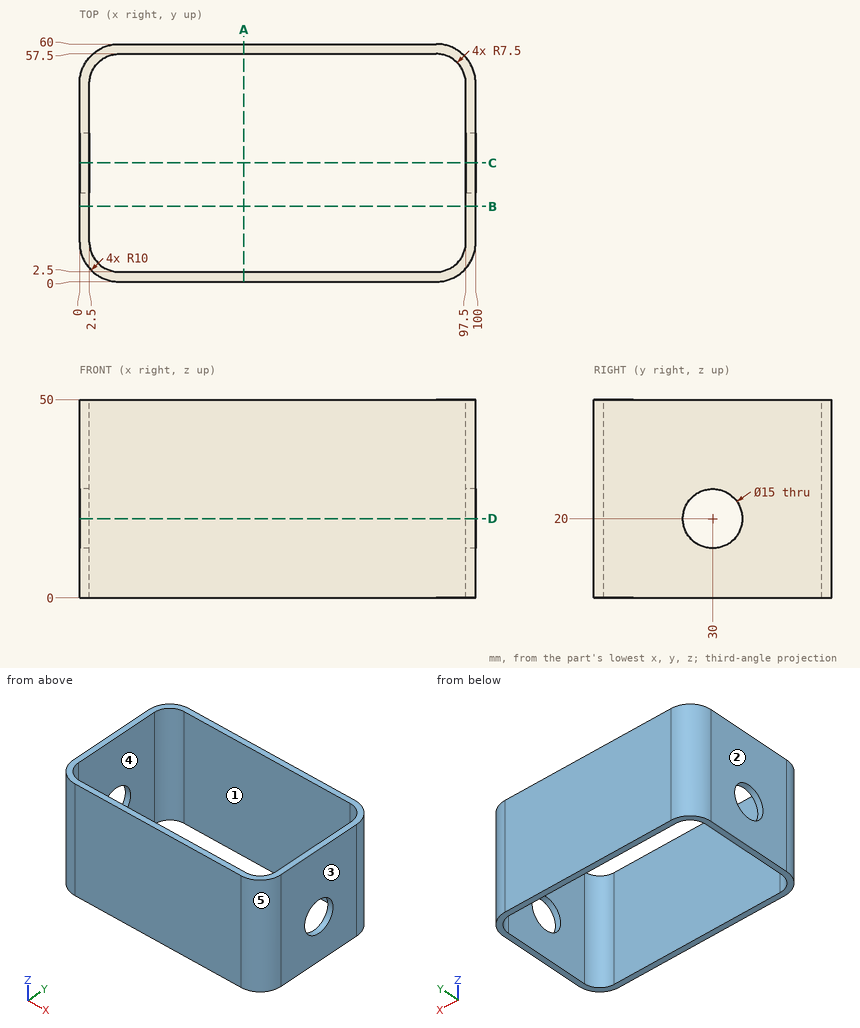
Input: dimensioned drawing with shaded views. Units: mm. Origin: part minimum x, y, z. A direction names the side the tool comes from. Give positions to 0.01 mm unless a question says otherwise; leave off trailing zeros. Loops run counter-clockwise (first coordinate to the right, second up) from the corner with the lowest first, then second, coordinate; pieces in that order, holes last. Notation, with made-up numbers: M 16.5,30.5 L 48.5,30.5 A16 ccw 48.5,47.5 Z; hole C -11.5,39 d3. An arc over 180 degrees is marked long. Put each result on its own line as item: value.
1) Cut plane C-C, the plane y = 30. Return the cut outline in (x, z), plus the area to 3 significant figures.
Computed values:
outline: M 0,0 L 2.5,0 L 2.5,12.5 L 0,12.5 Z; M 0,27.5 L 2.5,27.5 L 2.5,50 L 0,50 Z; M 97.5,0 L 100,0 L 100,12.5 L 97.5,12.5 Z; M 97.5,27.5 L 100,27.5 L 100,50 L 97.5,50 Z
area: 175 mm^2
2) Cut plane B-B, the plane y = 19. Return the cut outline in (x, z), plus the area to 3 significant figures.
Computed values:
outline: M 0,0 L 2.5,0 L 2.5,50 L 0,50 Z; M 97.5,0 L 100,0 L 100,50 L 97.5,50 Z
area: 250 mm^2
3) First-contact query: P1, Ø12, axis at y = 30, z = 20, coming from the +X side; P2, Ø5, axis at y = 6, z = 39.5, coming from the +X side. Flat tips, straight axial feed; report the tip coordinate or a pass-through.
Computed values:
P1: passes through
P2: stops at x = 99.89
4) Mould query, pull axis X, two halves, no side actions, for the marked faces 1, 2 and 3. Classes: released by +X, released by -X, zero draft, split by the parting line, or undercut.
Computed values:
face 1: undercut
face 2: released by -X
face 3: released by +X
5) Material intervals for L1, parallel to X at y = 13, z = 32; L2, parallel to Y at x = 62, z = 20; L3, parallel to Z at x = 99.15, y = 30, sorted ascending. Write a range as from..to.
Computed values:
L1: x = 0..2.5, 97.5..100
L2: y = 0..2.5, 57.5..60
L3: z = 0..12.5, 27.5..50
6) Reachability of the marked faces 4 and 5 from +Z, -Z, +X, -X, +Y, -Y: full face, straight path, thin tool, end or side. Return the list, or none.
Computed values:
face 4: +Z, -Z
face 5: +Z, -Z, +X, -Y
7) Cut plane A-A, the plane x = 41.5. Return the cut outline in (y, z).
Computed values:
outline: M 0,0 L 2.5,0 L 2.5,50 L 0,50 Z; M 57.5,0 L 60,0 L 60,50 L 57.5,50 Z
8) Cut plane D-D, the plane z = 20. Return the cut outline in (x, y), plus the area to 3 significant figures.
Computed values:
outline: M 0,10 A10 ccw 10,0 L 90,0 A10 ccw 100,10 L 100,22.5 L 97.5,22.5 L 97.5,10 A7.5 cw 90,2.5 L 10,2.5 A7.5 cw 2.5,10 L 2.5,22.5 L 0,22.5 Z; M 0,37.5 L 2.5,37.5 L 2.5,50 A7.5 cw 10,57.5 L 90,57.5 A7.5 cw 97.5,50 L 97.5,37.5 L 100,37.5 L 100,50 A10 ccw 90,60 L 10,60 A10 ccw 0,50 Z
area: 662 mm^2
